from build123d import *

# Parameters (mm, degrees)
SKETCH1_R           = 5
BOSS_EXTRUDE1_DEPTH = 8
SKETCH2_R           = 15
BOSS_EXTRUDE2_DEPTH = 12
SKETCH3_R           = 10
CUT_EXTRUDE1_DEPTH  = 21


with BuildPart() as part:
    # Sketch1 → Boss-Extrude1 (new body)
    with BuildSketch(Plane.XY):
        with BuildLine():
            Line((-9.871170143, 76.6), (-21.716574315, 3.52))
            ThreePointArc((-21.716574315, 3.52), (-15.360764468, -15.749505229), (4.061538462, -21.62183862))
            Line((4.061538462, -21.62183862), (66.846153846, -9.828108464))
            ThreePointArc((66.846153846, -9.828108464), (75, 0), (66.846153846, 9.828108464))
            Line((66.846153846, 9.828108464), (26.146237666, 17.473354451))
            ThreePointArc((26.146237666, 17.473354451), (20.833525499, 20.319297247), (18.121221369, 25.701462915))
            Line((18.121221369, 25.701462915), (9.871170143, 76.6))
            ThreePointArc((9.871170143, 76.6), (0, 85), (-9.871170143, 76.6))
        make_face()
        with Locations((0, 75)):
            Circle(SKETCH1_R, mode=Mode.SUBTRACT)
        with Locations((65, 0)):
            Circle(SKETCH1_R, mode=Mode.SUBTRACT)
    extrude(amount=BOSS_EXTRUDE1_DEPTH)

    # Sketch2 → Boss-Extrude2 (add)
    with BuildSketch(Plane.XY.offset(8)):
        Circle(SKETCH2_R)
    extrude(amount=BOSS_EXTRUDE2_DEPTH)

    # Sketch3 → Cut-Extrude1 (cut, through all)
    with BuildSketch(Plane.XY.offset(20)):
        Circle(SKETCH3_R)
    extrude(amount=-CUT_EXTRUDE1_DEPTH, mode=Mode.SUBTRACT)


solid = part.part
Input: part model. Units: mm. Frame: model coordinates. Coordinates: 2 decimals unless noted, no trailing zeros. Order: outer loops, then holes, each group sorted by start corner. A loop starts at its lowest first (then second) coordinate and runs counter-clockwise, first axis right, second up.
1. Ray query, line 1 along Y through (x, z) = (0, 2); line 2 along Y through (x, z) = (0, 14.75); line 3 along Z through (x, y) = (54.5, -12). Return the intervals inside material, ascending.
Checked values:
line 1: y = -22 to -10, 10 to 70, 80 to 85
line 2: y = -15 to -10, 10 to 15
line 3: z = 0 to 8
2. Cut plane D-D, the plane y = 75. Return loops of the section in (x, z).
Checked values:
outline: (-10.13, 0) - (-5, 0) - (-5, 8) - (-10.13, 8) - close; (5, 0) - (10.13, 0) - (10.13, 8) - (5, 8) - close
3. Cut plane B-B, the plane x = 0. Return loops of the section in (y, z), plus the area to 3 significant figures.
Checked values:
outline: (-22, 0) - (-10, 0) - (-10, 20) - (-15, 20) - (-15, 8) - (-22, 8) - close; (10, 0) - (70, 0) - (70, 8) - (15, 8) - (15, 20) - (10, 20) - close; (80, 0) - (85, 0) - (85, 8) - (80, 8) - close
area: 736 mm2
4. Contact query for flat-ended pins moving along their axis: P1, Ø11.5, axis at x = 0, y = 75, coming from the -Z side; P2, Ø5, axis at y = 20, z = 5, coming from the -X side; P3, Ø2, axis at x = -2, z = 5.5, coming from the +Y side; P4, Ø1.5, axis at y = 70, z = 4.5, coming from the -X side. Output: stop coordinate, or through.
Checked values:
P1: stops at z = 0
P2: stops at x = -19.45
P3: stops at y = 84.95
P4: stops at x = -11.06
5. Draft query along Y for faces 1 (the cylindrical face through (-14.985, 0.66, 13.916)), 2 (the cylindrical face through (20.89, 20.26, 3.94)), 3 (the cylindrical face through (-2.17, -9.76, 10.14)). Return one class per face: +Y half, -Y half, draft (parallel to the pull), parting line (faces both ways), or undercut.
Checked values:
face 1: parting line
face 2: +Y half
face 3: undercut
6. Cut plane A-A, the plane y = 0. Return loops of the section in (x, z).
Checked values:
outline: (-22, 0) - (-10, 0) - (-10, 20) - (-15, 20) - (-15, 8) - (-22, 8) - close; (10, 0) - (60, 0) - (60, 8) - (15, 8) - (15, 20) - (10, 20) - close; (70, 0) - (75, 0) - (75, 8) - (70, 8) - close
7. Cut plane C-C, the plane z = 6.25. Return loops of the section in (x, y), plus the area to 3 significant figures.
Checked values:
outline: (-21.72, 3.52) arc R22 ccw to (4.06, -21.62) - (66.85, -9.83) arc R10 ccw to (66.85, 9.83) - (26.15, 17.47) arc R10 cw to (18.12, 25.7) - (9.87, 76.6) arc R10 ccw to (-9.87, 76.6) - close; hole circle Ø20 at (0, 0); hole circle Ø10 at (0, 75); hole circle Ø10 at (65, 0)
area: 4,350 mm2
